```python
from build123d import *

# Parameters (mm, degrees)
RESSALTO_EXTRUS_O1_DEPTH = 1.6
RESSALTO_EXTRUS_O2_DEPTH = 1
CHANFRO1_SIZE            = 1
FILETE1_R                = 10


with BuildPart() as part:
    # Esboço1 → Ressalto-extrusão1 (new body)
    with BuildSketch(Plane.XY):
        with BuildLine():
            Line((0, 0), (50, 0))
            Line((50, 0), (50, -5))
            Line((50, -5), (75, -5))
            Line((75, -5), (75, 0))
            Line((75, 0), (61.5, 0))
            ThreePointArc((61.5, 0), (58.939339828, -1.060660172), (60, 1.5))
            Line((60, 1.5), (60, 10))
            Line((60, 10), (0, 10))
            Line((0, 10), (0, 0))
        make_face()
    extrude(amount=RESSALTO_EXTRUS_O1_DEPTH)

    # Esboço2 → Ressalto-extrusão2 (add)
    with BuildSketch(Plane.XY.offset(1.6)):
        Polygon((60, 7), (67, 0), (67, -5), (50, -5), (50, 7), align=None)
    extrude(amount=RESSALTO_EXTRUS_O2_DEPTH)

    # Chanfro1
    # the kernel refuses this chamfer: 1 mm, written as the material it adds along each edge
    with BuildSketch(Plane(origin=(50, 7, 1.6), x_dir=(0, 0.9996219169112968, -0.02749587661058627), z_dir=(1, 0, 0))) as chanfro1_piece_1_section:
        Polygon((CHANFRO1_SIZE * 0.999621916911, CHANFRO1_SIZE * 0.0274958766106), (-CHANFRO1_SIZE * 0.0274958766106, CHANFRO1_SIZE * 0.999621916911), (0, 0), align=None)
    chanfro1_piece_1 = extrude(amount=10, mode=Mode.PRIVATE)
    chanfro1_piece_1 = split(chanfro1_piece_1, bisect_by=Plane(origin=(57.256943657, 9.743056343, 1.932086514), z_dir=(-0.7071067811865478, -0.7071067811865474, 0)), keep=Keep.TOP, mode=Mode.PRIVATE)
    chanfro1_piece_1 = split(chanfro1_piece_1, bisect_by=Plane(origin=(54.837757031, 7.323869717, 2.6), z_dir=(0, 0, -1)), keep=Keep.TOP, mode=Mode.PRIVATE)
    add(chanfro1_piece_1)
    with BuildSketch(Plane(origin=(50, 7, 1.6), x_dir=(0, 0.9996219169112968, -0.02749587661058627), z_dir=(1, 0, 0))) as chanfro1_piece_2_section:
        Polygon((CHANFRO1_SIZE * 0.999621916911, CHANFRO1_SIZE * 0.0274958766106), (-CHANFRO1_SIZE * 0.0274958766106, CHANFRO1_SIZE * 0.999621916911), (0, 0), align=None)
    chanfro1_piece_2 = extrude(amount=10, mode=Mode.PRIVATE)
    chanfro1_piece_2 = split(chanfro1_piece_2, bisect_by=Plane(origin=(59.609036426, 7.390963574, 1.827791028), z_dir=(0.7071067811865478, 0.7071067811865474, 0)), keep=Keep.TOP, mode=Mode.PRIVATE)
    add(chanfro1_piece_2)
    with BuildSketch(Plane(origin=(50, 0, 1.6), x_dir=(-0.9996219169112968, 0, -0.0274958766105862), z_dir=(0, 1, 0))) as chanfro1_piece_3_section:
        Polygon((CHANFRO1_SIZE * 0.999621916911, CHANFRO1_SIZE * 0.0274958766106), (-CHANFRO1_SIZE * 0.0274958766106, CHANFRO1_SIZE * 0.999621916911), (0, 0), align=None)
    chanfro1_piece_3 = extrude(amount=7, mode=Mode.PRIVATE)
    chanfro1_piece_3 = split(chanfro1_piece_3, bisect_by=Plane(origin=(49.669595846, 3.5, 2.6), z_dir=(0, 0, -1)), keep=Keep.TOP, mode=Mode.PRIVATE)
    add(chanfro1_piece_3)
    with BuildSketch(Plane(origin=(67, 0, 1.6), x_dir=(0.9996219169112968, 0, -0.02749587661058639), z_dir=(0, -1, 0))) as chanfro1_piece_4_section:
        Polygon((CHANFRO1_SIZE * 0.999621916911, CHANFRO1_SIZE * 0.0274958766106), (-CHANFRO1_SIZE * 0.0274958766106, CHANFRO1_SIZE * 0.999621916911), (0, 0), align=None)
    chanfro1_piece_4 = extrude(amount=5, mode=Mode.PRIVATE)
    chanfro1_piece_4 = split(chanfro1_piece_4, bisect_by=Plane(origin=(67.390963574, -0.390963574, 1.827791028), z_dir=(0.7071067811865478, 0.7071067811865474, 0)), keep=Keep.TOP, mode=Mode.PRIVATE)
    add(chanfro1_piece_4)
    with BuildSketch(Plane(origin=(67, 0, 1.6), x_dir=(0.9996219169112968, 0, -0.02749587661058639), z_dir=(0, -1, 0))) as chanfro1_piece_5_section:
        Polygon((CHANFRO1_SIZE * 0.999621916911, CHANFRO1_SIZE * 0.0274958766106), (-CHANFRO1_SIZE * 0.0274958766106, CHANFRO1_SIZE * 0.999621916911), (0, 0), align=None)
    chanfro1_piece_5 = extrude(amount=5, mode=Mode.PRIVATE)
    chanfro1_piece_5 = split(chanfro1_piece_5, bisect_by=Plane(origin=(67.316872032, -2.658755048, 2.6), z_dir=(0, 0, -1)), keep=Keep.TOP, mode=Mode.PRIVATE)
    chanfro1_piece_5 = split(chanfro1_piece_5, bisect_by=Plane(origin=(68.48781354, -1.48781354, 1.93578343), z_dir=(-0.7071067811865478, -0.7071067811865474, 0)), keep=Keep.TOP, mode=Mode.PRIVATE)
    add(chanfro1_piece_5)
    with BuildSketch(Plane(origin=(47.428317012, 7, 1.6), x_dir=(0, 0.9996219169112968, -0.02749587661058627), z_dir=(1, 0, 0))) as chanfro1_piece_6a_section:
        Polygon((CHANFRO1_SIZE * 0.999621916911, CHANFRO1_SIZE * 0.0274958766106), (-CHANFRO1_SIZE * 0.0274958766106, CHANFRO1_SIZE * 0.999621916911), (0, 0), align=None)
    chanfro1_piece_6a = extrude(amount=12.571682988, mode=Mode.PRIVATE)
    chanfro1_piece_6a = split(chanfro1_piece_6a, bisect_by=Plane(origin=(50, 7.330404154, 1.928634334), z_dir=(-1, 0, 0)), keep=Keep.TOP, mode=Mode.PRIVATE)
    chanfro1_piece_6a = split(chanfro1_piece_6a, bisect_by=Plane(origin=(48.714158506, 7.330404154, 2.6), z_dir=(0, 0, -1)), keep=Keep.TOP, mode=Mode.PRIVATE)
    with BuildSketch(Plane(origin=(50, 0, 1.6), x_dir=(-0.9996219169112968, 0, -0.0274958766105862), z_dir=(0, 1, 0))) as chanfro1_piece_6b_section:
        Polygon((CHANFRO1_SIZE * 0.999621916911, CHANFRO1_SIZE * 0.0274958766106), (-CHANFRO1_SIZE * 0.0274958766106, CHANFRO1_SIZE * 0.999621916911), (0, 0), align=None)
    chanfro1_piece_6b = extrude(amount=9.571682988, mode=Mode.PRIVATE)
    chanfro1_piece_6b = split(chanfro1_piece_6b, bisect_by=Plane(origin=(49.669595846, 7, 1.928634334), z_dir=(0, 1, 0)), keep=Keep.TOP, mode=Mode.PRIVATE)
    chanfro1_piece_6b = split(chanfro1_piece_6b, bisect_by=Plane(origin=(49.669595846, 8.285841494, 2.6), z_dir=(0, 0, -1)), keep=Keep.TOP, mode=Mode.PRIVATE)
    chanfro1_piece_6 = chanfro1_piece_6a & chanfro1_piece_6b
    add(chanfro1_piece_6)

    # Filete1
    filete1_edges = [part.edges().sort_by_distance(p)[0] for p in [
        (60, 1.5, 0.8),
        (61.5, 0, 0.8),
    ]]
    fillet(filete1_edges, radius=FILETE1_R)


solid = part.part
```
For this review, take the finished solid that the model builds, in its own axes (mm). A direction names the side the tool comes from. Give positions to 0.01 mm unless a question says otherwise; leave off trailing zeros. Write each loop counter-clockwise with the first axis right and the second up, starting at its lowest first coordinate (ties: lowest second). Pieces come first, ordered by that corner, then holes. Notation, with made-up numbers: M -37.75,44 L -10.75,44 A30 ccw -10.75,74 Z; hole C 16,27 d10. An arc over 180 degrees is marked long. Answer as a JSON object with one key per item and string values. Group by question number.
Item 1: For pin 1 Ø1.5 at (y, z) = (5, 0.5) entering from +X; pin 2 Ø1.3 at (y, z) = (-3.5, 1.5) entering from -X; pin 3 Ø8 at (x, y) = (30.5, 4.5) entering from +Z, all flat-tipped, find the tip position at first contact; note any pin that passes through.
Item 2: Draft analysis for pull direction X (two halves, no side actions). For faces 6 (the flat face through (60, 8, 1)), 7 (the flat face through (37, 4, 0)), 8 (the flat face through (62, 2, 1.6)), state which applies: +X half, -X half, draft (parallel to the pull), parting line (faces both ways), or undercut.
Item 3: Consider section B-B on y = 1.75. Write out the cut boundary in (x, z).
Item 4: Consider section A-A on z = 0.95. Write out the cut boundary in (x, y).
Item 5: For probe 1 along X at (y, z) = (7.25, 0.4); probe 2 along Y at (x, z) = (67.5, 1.9); probe 3 along Y at (x, z) = (6, 0.1), list the stretches that pass through material, from the lowest coordinate up. Write a range as [from, to].
Item 6: Consider section C-C on x = 19. Write out the cut boundary in (y, z), plus the area to 3 significant figures.
Item 7: Tool access review of faces 1 (the cylindrical face through (59.66, 3.09, 0.81)), 2 (the flat face through (50, -3, 1)), 3 (the cylindrical face through (58.96, -1.08, 0.79)), 4 (the cylindrical face through (63.09, -0.34, 0.81)), 5 (the flat face through (71, -2, 1.6)): name each direction out of +Z, -Z, +X, -X, +Y, -Y from which nothing blocks a thin tool from reaching the whole face with its end or side.
Item 8: Consider section D-D on y = -3.75. Write out the cut boundary in (x, z).
Check result:
{
 "1": {"pin 1": "stops at x = 60", "pin 2": "stops at x = 50", "pin 3": "stops at z = 1.6"},
 "2": {"face 6": "+X half", "face 7": "draft", "face 8": "undercut"},
 "3": {"outline": "M 0,0 L 59.2,0 L 59.2,1.6 L 65.25,1.6 L 65.25,2.6 L 50,2.6 L 49,1.6 L 0,1.6 Z"},
 "4": {"outline": "M 0,0 L 50,0 L 50,-5 L 75,-5 L 75,0 L 65.68,0 A10 ccw 60.74,-1.3 A1.5 cw 58.7,0.74 A10 ccw 60,5.68 L 60,10 L 0,10 Z"},
 "5": {"probe 1": "x = [0, 60]", "probe 2": "y = [-5, 0]", "probe 3": "y = [0, 10]"},
 "6": {"outline": "M 0,0 L 10,0 L 10,1.6 L 0,1.6 Z", "area": "16.0 mm^2"},
 "7": {"face 1": "-Z, +X", "face 2": "+Z, -Z, -X, -Y", "face 3": "-Z", "face 4": "-Z, +Y", "face 5": "+Z, +X, +Y, -Y"},
 "8": {"outline": "M 50,0 L 75,0 L 75,1.6 L 68,1.6 L 67,2.6 L 50,2.6 Z"}
}
